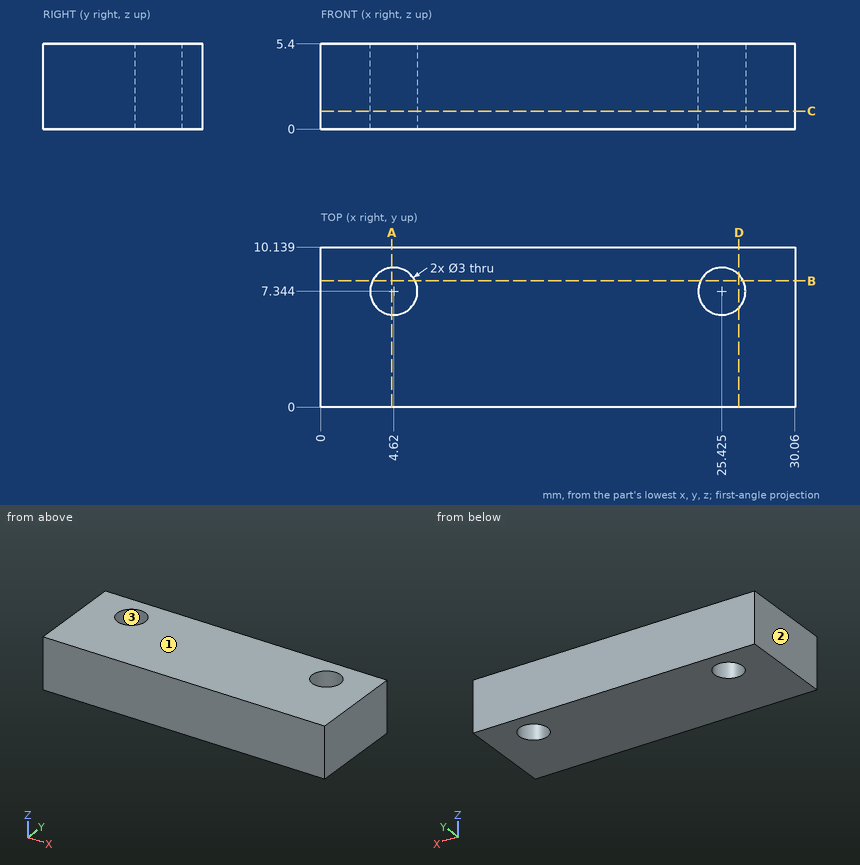
Could you check a few things on this drawing? It's one solid part, dimensions in mm from its lowest x, y, z. Round coordinates to 2 decimals unless told otherwise and drop trailing zeros. Write each loop counter-clockwise with the first axis right and the second up, starting at its lowest first coordinate (ties: lowest second). Pieces come first, ordered by that corner, then holes. Notation, with made-up numbers: (34.5, -1) -> (52.5, -1) arc R20 ccw to (52.5, 37) -> close; hole circle Ø10 at (1, 35). An arc over 180 degrees is marked (long way). One line per question, with ' | ' between items. Start each with the question number.
1) If we mould it in two halves opening along X, with no side actions, what happens to the marked faces 1, 2 and 3? For each: released by +X, released by -X, zero draft, split by the parting line, or undercut.
2) Suppose I cut it at A-A on x = 4.5. Write out the boundary of the cut face in (y, z).
3) I need wall thicknesses on line 1 (Y direction, x = 4.5, z = 5.15); line 2 (Y direction, x = 24.5, z = 5.1) (1 decimal). Which ranges of each line are inside material? Lowest first, please. Write a range as [from, to].
4) Suppose I cut it at D-D on x = 26.5. Write out the boundary of the cut face in (y, z).
5) Suppose I cut it at C-C on z = 1.15. Write out the boundary of the cut face in (x, y) (1 decimal), then the cut area to 3 significant figures.
6) Suppose I cut it at B-B on y = 8. Write out the boundary of the cut face in (x, z) (1 decimal).
Return value:
1) face 1: zero draft | face 2: released by -X | face 3: undercut
2) outline: (0, 0) -> (5.85, 0) -> (5.85, 5.4) -> (0, 5.4) -> close; (8.84, 0) -> (10.14, 0) -> (10.14, 5.4) -> (8.84, 5.4) -> close
3) line 1: y = [0, 5.85], [8.84, 10.14] | line 2: y = [0, 6.2], [8.5, 10.1]
4) outline: (0, 0) -> (6.3, 0) -> (6.3, 5.4) -> (0, 5.4) -> close; (8.39, 0) -> (10.14, 0) -> (10.14, 5.4) -> (8.39, 5.4) -> close
5) outline: (0, 0) -> (30.1, 0) -> (30.1, 10.1) -> (0, 10.1) -> close; hole circle Ø3 at (4.6, 7.3); hole circle Ø3 at (25.4, 7.3) | area: 291 mm2
6) outline: (0, 0) -> (3.3, 0) -> (3.3, 5.4) -> (0, 5.4) -> close; (6, 0) -> (24.1, 0) -> (24.1, 5.4) -> (6, 5.4) -> close; (26.8, 0) -> (30.1, 0) -> (30.1, 5.4) -> (26.8, 5.4) -> close
